Autodesk Inventor part; units mm, degrees
ref_plane "YZ Plane" through (0, 0, 0) normal (1, 0, 0) x (0, 1, 0)
ref_plane "XZ Plane" through (0, 0, 0) normal (0, 1, 0) x (-1, 0, 0)
ref_plane "XY Plane" through (0, 0, 0) normal (0, 0, 1) x (1, 0, 0)
sketch "Sketch1" plane through (0, 0, 0) normal (0, 1, 0) x (-1, 0, 0)
  line L0 (0, 0) -> (30, 0)
  line L1 (30, 0) -> (30, -3)
  line L2 (30, -3) -> (0, -3)
  line L3 (0, -3) -> (0, 0)
  dimension "d0" = 30
  dimension "d1" = 3
extrude "Extrusion1" add sketch "Sketch1" along normal blind 7.5
sketch "Sketch2" plane through (0, 7.5, 0) normal (0, 1, 0) x (1, 0, 0)
  circle A0 centre (-1.8095, 1.2925) radius 0.9997
  point P0 (0, 0)
extrude "Extrusion2" cut sketch "Sketch2" against normal blind 0.1
sketch "Sketch3" plane through (-30, 0, 0) normal (0, 0, 1) x (1, 0, 0)
  circle A0 centre (26.5, 2.5) radius 0.6105
  circle A1 centre (22, 2.5) radius 1.95
  circle A2 centre (17.5, 2.5) radius 0.6105
  line L0 (0, 0) -> (30, 0)
  line L1 (30, 0) -> (30, 7.5)
  line L2 (0, 7.5) -> (30, 7.5)
  line L3 (0, 7.5) -> (30, 7.5)
  line L4 (30, 7.5) -> (15, 7.5)
  line L5 (15, 0) -> (15, 7.5)
  circle A3 centre (3.5, 2.5) radius 0.6105
  circle A4 centre (8, 2.5) radius 1.95
  circle A5 centre (12.5, 2.5) radius 0.6105
  dimension "d6" = 1.221
  dimension "d7" = 3.9
  dimension "d8" = 1.221
  dimension "d9" = 2.5
  dimension "d10" = 2.5
  dimension "d11" = 2.5
  dimension "d12" = 3.5
  dimension "d13" = 8
  dimension "d14" = 4.5
extrude "Extrusion3" cut sketch "Sketch3" against normal blind 3 contours A0 | A1 | A2 | A3 | A4 | A5
properties part number "backmidmotorwall"
Here's how the part is built. I have some questions about the finished solid (model axes, mm). Give positions to 0.01 mm unless a question says otherwise; leave off trailing zeros. Order: outer loops, then holes, each group sorted by start corner. A loop starts at its lowest first (then second) coordinate and runs counter-clockwise, first axis right, second up. Notation, with made-up numbers: M 35.5,4 L 72.5,4 A20 cw 72.5,12 Z; hole C -1.75,31 d4. An arc over 180 degrees is marked long. Use a Markdown table: item, result. Add a question column.
1. Suppose I cut it at A-A (y = 2.5). List the corners of the cut face in (x, z) for me.
2. Suppose I cut it at C-C (z = -2.55). List the corners of the cut face in (x, y) for me.
3. If we mould it in two halves opening along Y, with no side actions, what happens to faces 1 (the cylindrical face through (-12.172, 3.015, -1.479)), 2 (the flat face through (-15, 4, 0)), 3 (the flat face through (-2, 7.4, -1))? For each: +Y half, -Y half, draft (parallel to the pull), parting line (faces both ways), or undercut.
4. For pin 1 Ø4.5 at (x, y) = (-22, 2.5) entering from +Z; pin 2 Ø1 at (x, z) = (-1.5, -1) entering from +Y; pin 3 Ø1 at (x, y) = (-17.5, 2.5) entering from +Z, each with a flat end and sliding along its axis, tell me the tip position at first contact or that it passes through.
5. Suppose I cut it at D-D (y = 3.75). List the corners of the cut face in (x, z) for me.
6. Suppose I cut it at B-B (x = -3.5). List the corners of the cut face in (y, z) for me, and give its area (3 significant figures).
7. I need wall thicknesses on probe 1 along Y at (x, z) = (-8, -1.7); probe 2 along Y at (x, z) = (-3.5, -0.95); probe 3 along X at (y, z) = (1, -1.55). Which ranges of each line are inside material? Lowest first, please. Write a range as from..to.
Results list:
| question | item | result |
|---|---|---|
| 1 | outline | M -30,-3 L -27.11,-3 L -27.11,0 L -30,0 Z; M -25.89,-3 L -23.95,-3 L -23.95,0 L -25.89,0 Z; M -20.05,-3 L -18.11,-3 L -18.11,0 L -20.05,0 Z; M -16.89,-3 L -13.11,-3 L -13.11,0 L -16.89,0 Z; M -11.89,-3 L -9.95,-3 L -9.95,0 L -11.89,0 Z; M -6.05,-3 L -4.11,-3 L -4.11,0 L -6.05,0 Z; M -2.89,-3 L 0,-3 L 0,0 L -2.89,0 Z |
| 2 | outline | M -30,0 L 0,0 L 0,7.5 L -30,7.5 Z; hole C -26.5,2.5 d1.22; hole C -22,2.5 d3.9; hole C -17.5,2.5 d1.22; hole C -12.5,2.5 d1.22; hole C -8,2.5 d3.9; hole C -3.5,2.5 d1.22 |
| 3 | face 1 | undercut |
| 3 | face 2 | draft |
| 3 | face 3 | +Y half |
| 4 | pin 1 | stops at z = 0 |
| 4 | pin 2 | stops at y = 7.4 |
| 4 | pin 3 | passes through |
| 5 | outline | M -30,-3 L -23.5,-3 L -23.5,0 L -30,0 Z; M -20.5,-3 L -9.5,-3 L -9.5,0 L -20.5,0 Z; M -6.5,-3 L 0,-3 L 0,0 L -6.5,0 Z |
| 6 | outline | M 0,-3 L 1.89,-3 L 1.89,0 L 0,0 Z; M 3.11,-3 L 7.5,-3 L 7.5,0 L 3.11,0 Z |
| 6 | area | 18.8 mm² |
| 7 | probe 1 | y = 0..0.55, 4.45..7.5 |
| 7 | probe 2 | y = 0..1.89, 3.11..7.5 |
| 7 | probe 3 | x = -30..-23.25, -20.75..-9.25, -6.75..0 |
